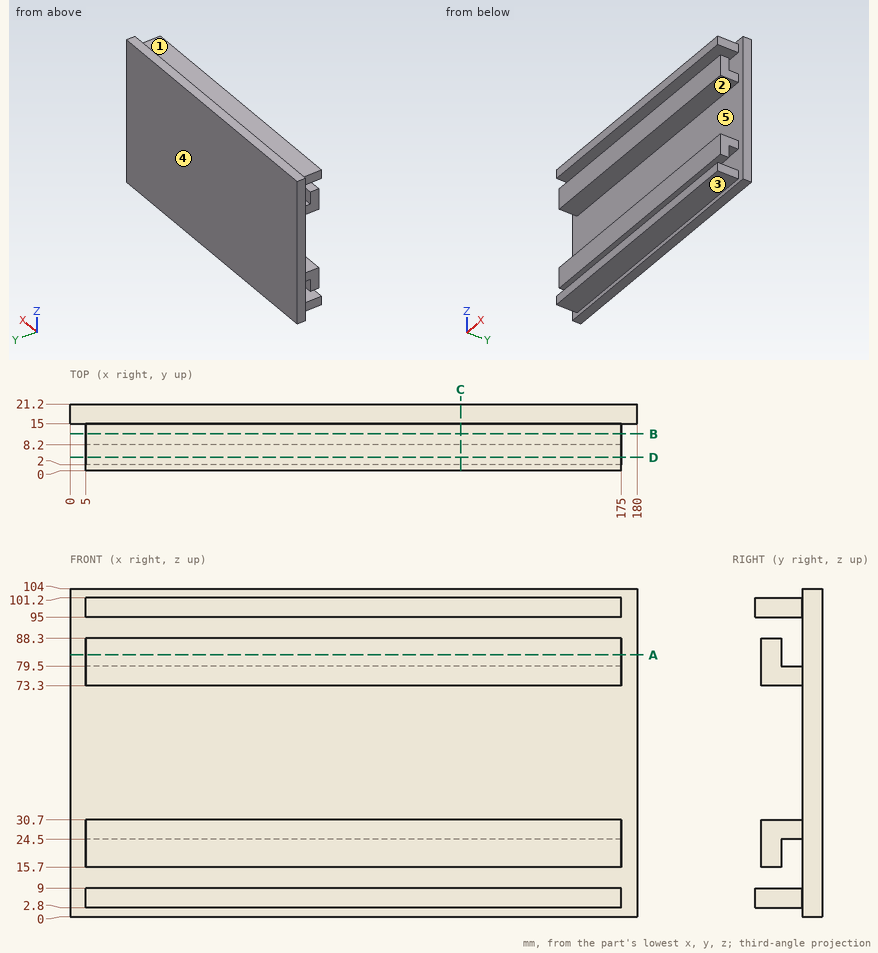
Part print with two shaded views. Sizes in mm from the minimum x, y, z corner. A direction names the side the tool comes from. Round coordinates to 2 decimals unless told otherwise and drop trailing zeros. Order: outer loops, then holes, each group sorted by start corner. A loop starts at its lowest first (then second) coordinate and runs counter-clockwise, first axis right, second up. Notation, with made-up numbers: M -25,10 L -3,10 A33 cw -3,44 Z; hole C -12,-15.75 d1. An arc over 180 degrees is marked long. Put each result on its own line as item: value. Start each with the question number.
1. Drill centre lines: probe 1 along Z at (x, y) = (28.5, 8); probe 2 along Z at (x, y) = (55, 12); probe 3 along Y at (x, z) = (155, 81.5). Where is each one in solid material? Low to high. Write a range as [from, to].
2. Two-plate mould, pull along Y, no slides. Class the marked faces 3, 4 and 5: +Y half, -Y half, draft (parallel to the pull), parting line (faces both ways), or undercut.
3. Tool access for the marked faces 1 and 2: list every direction of +Z, -Z, +X, -X, +Y, -Y with a clear straight run to the whole face (end or side of a thin tool).
4. Slice it at A-A on z = 83. List the corners of the cut face in (x, y).
5. Slice it at D-D on y = 4.25. List the corners of the cut face in (x, z), then the cut area to 3 significant figures.
6. Slice it at C-C on x = 124. List the corners of the cut face in (y, z), then the cut area to 3 significant figures.
7. Drop flat-ended pins along their axis: pin 1 (3 mm diameter, centred on x = 117.5, y = 12, fed in from +Z); pin 2 (4 mm diameter, centred on y = 8.5, z = 23, fed in from +X); pin 3 (7.5 mm diameter, centred on x = 97, z = 22.5, fed in from -Y); pin 4 (4 mm diameter, centred on y = 10.5, z = 84, fed in from -X). Give the stop position or say it passes through.
8. Slice it at B-B on y = 11.75. List the corners of the cut face in (x, z).
Findings:
1. probe 1: [2.8, 9], [15.7, 30.7], [73.3, 88.3], [95, 101.2]
1. probe 2: [2.8, 9], [24.5, 30.7], [73.3, 79.5], [95, 101.2]
1. probe 3: [2, 8.2], [15, 21.2]
2. face 3: draft
2. face 4: +Y half
2. face 5: undercut
3. face 1: +Z, +X, -X, -Y
3. face 2: +X, -X, -Y
4. outline: M 0,15 L 180,15 L 180,21.2 L 0,21.2 Z; M 5,2 L 175,2 L 175,8.2 L 5,8.2 Z
5. outline: M 5,2.8 L 175,2.8 L 175,9 L 5,9 Z; M 5,15.7 L 175,15.7 L 175,30.7 L 5,30.7 Z; M 5,73.3 L 175,73.3 L 175,88.3 L 5,88.3 Z; M 5,95 L 175,95 L 175,101.2 L 5,101.2 Z
5. area: 7,210 mm2
6. outline: M 0,2.8 L 15,2.8 L 15,0 L 21.2,0 L 21.2,104 L 15,104 L 15,101.2 L 0,101.2 L 0,95 L 15,95 L 15,79.5 L 8.2,79.5 L 8.2,88.3 L 2,88.3 L 2,73.3 L 15,73.3 L 15,30.7 L 2,30.7 L 2,15.7 L 8.2,15.7 L 8.2,24.5 L 15,24.5 L 15,9 L 0,9 Z
6. area: 1,100 mm2
7. pin 1: z = 101.2
7. pin 2: x = 175
7. pin 3: y = 2
7. pin 4: through
8. outline: M 5,2.8 L 175,2.8 L 175,9 L 5,9 Z; M 5,24.5 L 175,24.5 L 175,30.7 L 5,30.7 Z; M 5,73.3 L 175,73.3 L 175,79.5 L 5,79.5 Z; M 5,95 L 175,95 L 175,101.2 L 5,101.2 Z
